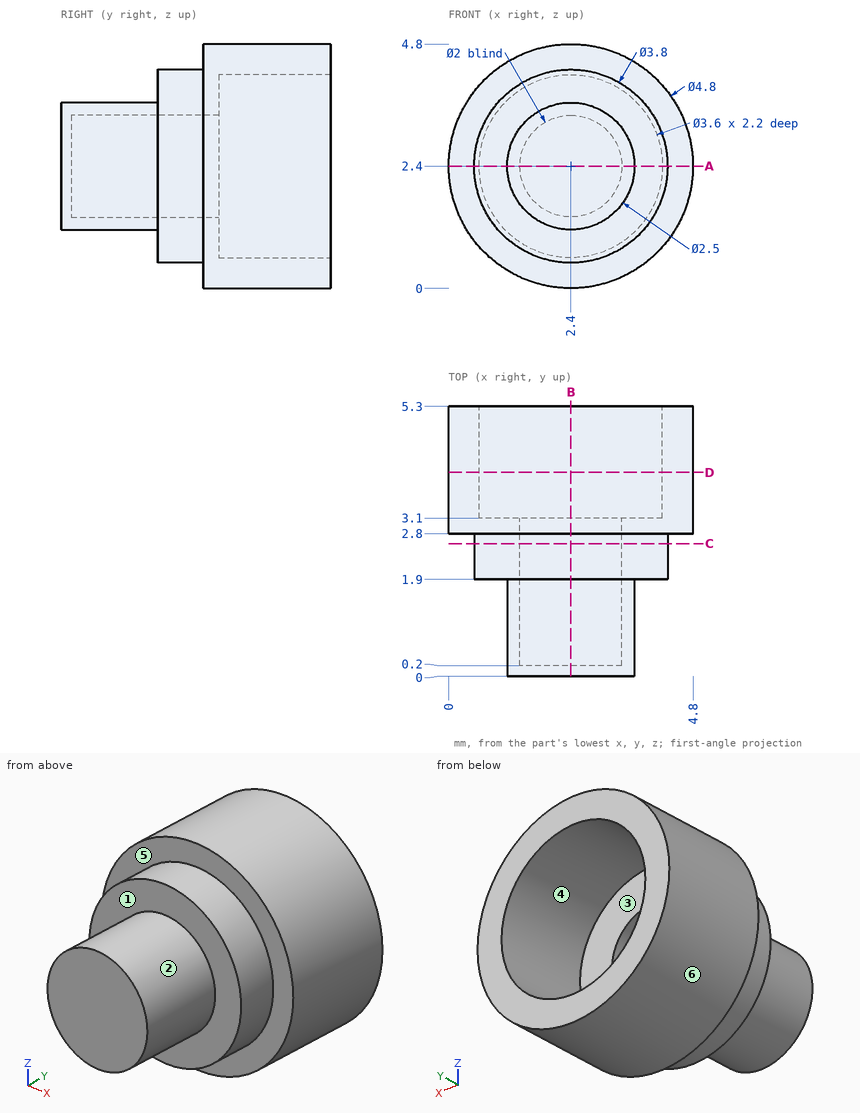
The drawing under review shows one solid part. Ordinate dimensions are in mm from its lowest x, y, z. A direction names the side the tool comes from. Round coordinates to 2 decimals unless told otherwise and drop trailing zeros. Write each loop counter-clockwise with the first axis right and the second up, starting at its lowest first coordinate (ties: lowest second). Pieces come first, ordered by that corner, then holes.
(1) We need section B-B on x = 2.4. Give the boundary of the cut face in (y, z), and give its area (3 significant figures).
(2) Mouldability with a two-part tool opening along Z and no side actions: class the marked faces 1, 2 and 3 as +Z half, -Z half, draft (parallel to the pull), parting line (faces both ways), or undercut.
(3) We need section D-D on y = 4. Give the boundary of the cut face in (x, z).
(4) Wall thickness on L1, parallel to X at y = 2.2, z = 2.4; L2, parallel to Y at x = 2.15, z = 3.5; L3, parallel to Y at x = 0.8, z = 1.25: over which ranges is each line inside the solid? List them lowest first.
(5) Machinability: for the marked faces 4, 5 and 6, which of the approach directions +Z, -Z, +X, -X, +Y, -Y give a long, thin tool a straight path to every point of the face, cutting with its end or side? Answer none if there is none.
(6) We need section C-C on y = 2.6. Give the boundary of the cut face in (x, z).
(7) We need section A-A on z = 2.4. Give the boundary of the cut face in (x, y).
(8) Insertion check: pin 1 (2 mm diameter, centred on x = 2.5, z = 2, fed in from +Y); pin 2 (1.1 mm diameter, centred on x = 2.5, z = 2, fed in from +Y); pin 3 (1 mm diameter, centred on x = 1, y = 1, fed in from -Z). Each pin has a flat end and moves straight along its axis. Give the tip position at first contact, or say it passes through.
Findings below:
1. outline: (0, 1.15) - (1.9, 1.15) - (1.9, 0.5) - (2.8, 0.5) - (2.8, 0) - (5.3, 0) - (5.3, 0.6) - (3.1, 0.6) - (3.1, 1.4) - (0.2, 1.4) - (0.2, 3.4) - (3.1, 3.4) - (3.1, 4.2) - (5.3, 4.2) - (5.3, 4.8) - (2.8, 4.8) - (2.8, 4.3) - (1.9, 4.3) - (1.9, 3.65) - (0, 3.65) - close
1. area: 6.45 mm2
2. face 1: draft
2. face 2: parting line
2. face 3: undercut
3. outline: circle Ø4.8 at (2.4, 2.4); hole circle Ø3.6 at (2.4, 2.4)
4. L1: x = 0.5 to 1.4, 3.4 to 4.3
4. L2: y = 0 to 3.1
4. L3: y = 2.8 to 5.3
5. face 4: +Y
5. face 5: -Y
5. face 6: +Y, -Y
6. outline: circle Ø3.8 at (2.4, 2.4); hole circle Ø2 at (2.4, 2.4)
7. outline: (0, 2.8) - (0.5, 2.8) - (0.5, 1.9) - (1.15, 1.9) - (1.15, 0) - (3.65, 0) - (3.65, 1.9) - (4.3, 1.9) - (4.3, 2.8) - (4.8, 2.8) - (4.8, 5.3) - (4.2, 5.3) - (4.2, 3.1) - (3.4, 3.1) - (3.4, 0.2) - (1.4, 0.2) - (1.4, 3.1) - (0.6, 3.1) - (0.6, 5.3) - (0, 5.3) - close
8. pin 1: stops at y = 3.1
8. pin 2: stops at y = 0.2
8. pin 3: stops at z = 1.53
